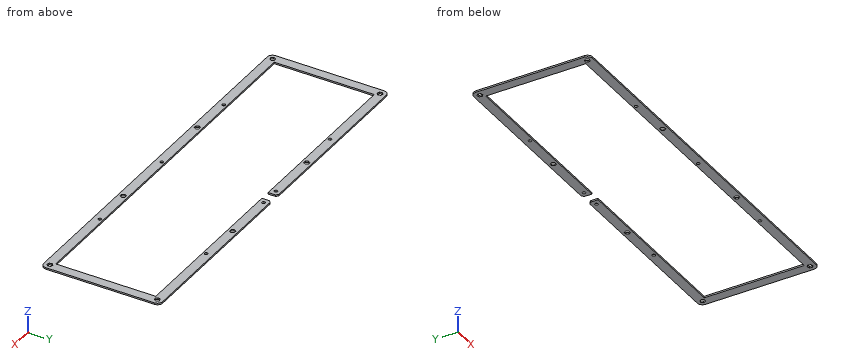
```python
from build123d import *

# Parameters (mm, degrees)
MODEL_R             = 1.55
BOSS_EXTRUDE1_DEPTH = 1.5


with BuildPart() as part:
    # Model → Boss-Extrude1 (new body)
    with BuildSketch(Plane.XY):
        with BuildLine():
            Line((0, 108.6), (0, 5))
            ThreePointArc((0, 5), (1.464466094, 1.464466094), (5, 0))
            Line((5, 0), (365.775, 0))
            ThreePointArc((365.775, 0), (369.310533906, 1.464466094), (370.775, 5))
            Line((370.775, 5), (370.775, 108.6))
            ThreePointArc((370.775, 108.6), (369.310533906, 112.135533906), (365.775, 113.6))
            Line((365.775, 113.6), (192.3875, 113.6))
            Line((192.3875, 113.6), (190.3875, 111.6))
            Line((190.3875, 111.6), (190.3875, 104.6))
            Line((190.3875, 104.6), (361.775, 104.6))
            Line((361.775, 104.6), (361.775, 9))
            Line((361.775, 9), (9, 9))
            Line((9, 9), (9, 104.6))
            Line((9, 104.6), (180.3875, 104.6))
            Line((180.3875, 104.6), (180.3875, 111.6))
            Line((180.3875, 111.6), (178.3875, 113.6))
            Line((178.3875, 113.6), (5, 113.6))
            ThreePointArc((5, 113.6), (1.464466094, 112.135533906), (0, 108.6))
        make_face()
        with Locations((195.3875, 109.1)):
            Circle(MODEL_R, mode=Mode.SUBTRACT)
        with Locations((175.3875, 109.1)):
            Circle(MODEL_R, mode=Mode.SUBTRACT)
        with Locations((85.3875, 107.6)):
            Circle(MODEL_R, mode=Mode.SUBTRACT)
        with Locations((285.3875, 107.6)):
            Circle(MODEL_R, mode=Mode.SUBTRACT)
        with Locations((85.3875, 6)):
            Circle(MODEL_R, mode=Mode.SUBTRACT)
        with Locations((185.3875, 6)):
            Circle(MODEL_R, mode=Mode.SUBTRACT)
        with Locations((285.3875, 6)):
            Circle(MODEL_R, mode=Mode.SUBTRACT)
        Polygon((365.947431604, 110.609548911), (367.784548911, 108.772431604), (367.112117307, 106.262882693), (364.602568396, 105.590451089), (362.765451089, 107.427568396), (363.437882693, 109.937117307), align=None, mode=Mode.SUBTRACT)
        Polygon((4.827568396, 110.609548911), (2.990451089, 108.772431604), (3.662882693, 106.262882693), (6.172431604, 105.590451089), (8.009548911, 107.427568396), (7.337117307, 109.937117307), align=None, mode=Mode.SUBTRACT)
        Polygon((365.947431604, 2.990451089), (367.784548911, 4.827568396), (367.112117307, 7.337117307), (364.602568396, 8.009548911), (362.765451089, 6.172431604), (363.437882693, 3.662882693), align=None, mode=Mode.SUBTRACT)
        Polygon((4.827568396, 2.990451089), (2.990451089, 4.827568396), (3.662882693, 7.337117307), (6.172431604, 8.009548911), (8.009548911, 6.172431604), (7.337117307, 3.662882693), align=None, mode=Mode.SUBTRACT)
        Polygon((243.975961894, 2.25), (246.574038106, 2.25), (247.873076211, 4.5), (246.574038106, 6.75), (243.975961894, 6.75), (242.676923789, 4.5), align=None, mode=Mode.SUBTRACT)
        Polygon((243.975961894, 106.85), (246.574038106, 106.85), (247.873076211, 109.1), (246.574038106, 111.35), (243.975961894, 111.35), (242.676923789, 109.1), align=None, mode=Mode.SUBTRACT)
        Polygon((124.200961894, 106.85), (126.799038106, 106.85), (128.098076211, 109.1), (126.799038106, 111.35), (124.200961894, 111.35), (122.901923789, 109.1), align=None, mode=Mode.SUBTRACT)
        Polygon((124.200961894, 2.25), (126.799038106, 2.25), (128.098076211, 4.5), (126.799038106, 6.75), (124.200961894, 6.75), (122.901923789, 4.5), align=None, mode=Mode.SUBTRACT)
    extrude(amount=BOSS_EXTRUDE1_DEPTH)


solid = part.part
```
Can you work these out from the model? Positions are in its coordinate system, mm. Coordinates: 2 decimals unless noted, no trailing zeros. Loops run counter-clockwise (first coordinate to the right, second up) from the corner with the lowest first, then second, coordinate; pieces in that order, holes last.
1) Imagine slicing it at C-C on z = 1.2. State how many separate pieces and enclosed holes the cut face has, plus the area to 3 significant figures.
2) Imagine slicing it at A-A on x = 42. List the corners of the cut face in (y, z) for me, plus the area to 3 significant figures.
3) I need wall thicknesses on probe 1 along Y at (x, z) = (285, 0.5); probe 2 along Y at (x, z) = (245, 0.4); probe 3 along X at (y, z) = (77.5, 0.75) (3 decimals). Which ranges of each line are inside material? Lowest first, please.
4) For pin 1 (3.5 mm diameter, centred on x = 175.39, y = 109.1, fed in from -Z), with a flat end and sliding along its axis, tell me the tip position at first contact or that it passes through.
5) Imagine slicing it at B-B on y = 24. List the corners of the cut face in (x, z) for me (3 decimals), plus the area to 3 significant figures.
Completed:
1. separate pieces: 1
1. enclosed holes: 15
1. area: 8,090 mm2
2. outline: (0, 0) - (9, 0) - (9, 1.5) - (0, 1.5) - close; (104.6, 0) - (113.6, 0) - (113.6, 1.5) - (104.6, 1.5) - close
2. area: 27.0 mm2
3. probe 1: y = 0 to 4.5, 7.5 to 9, 104.6 to 106.1, 109.1 to 113.6
3. probe 2: y = 0 to 2.25, 6.75 to 9, 104.6 to 106.85, 111.35 to 113.6
3. probe 3: x = 0 to 9, 361.775 to 370.775
4. pin 1: stops at z = 0
5. outline: (0, 0) - (9, 0) - (9, 1.5) - (0, 1.5) - close; (361.775, 0) - (370.775, 0) - (370.775, 1.5) - (361.775, 1.5) - close
5. area: 27.0 mm2
